Job drawing, mm, ordinate dimensions from the low corner. One solid piece. Round coordinates to 2 decimals unless told otherwise and drop trailing zeros. Loops run counter-clockwise (first coordinate to the right, second up) from the corner with the lowest first, then second, coordinate; pieces in that order, holes last. Notation, with made-up numbers: (-18, -19.5) - (30, -19.5) arc R16 cw to (30, 8.5) - close; hole circle Ø4 at (15, 37.25). An arc over 180 degrees is marked (long way). One line per question, with ' | ' between items. Start each with the question number.
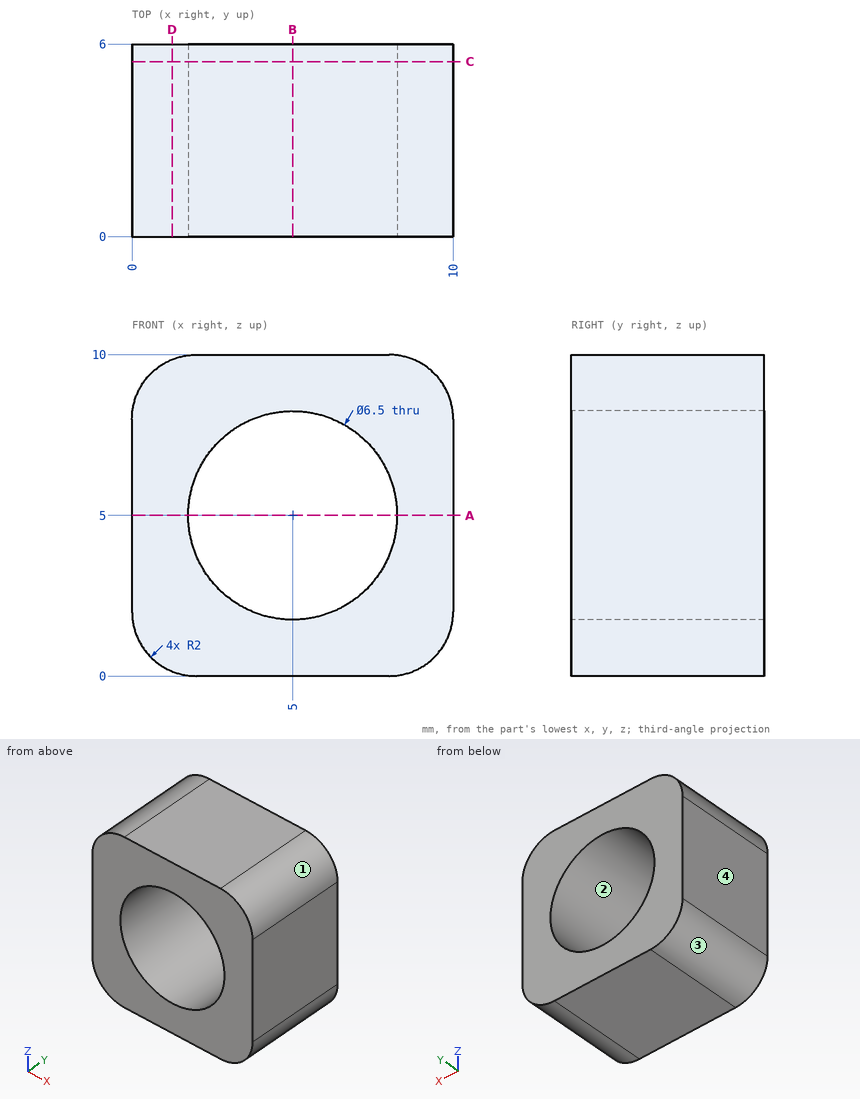
1) Saw through at B-B on x = 5. Write the cut outline in (y, z), and give its area (3 significant figures).
2) Saw through at A-A on z = 5. Write the cut outline in (x, y).
3) Saw through at D-D on x = 1.25. Write the cut outline in (y, z), and give its area (3 significant figures).
4) Saw through at C-C on y = 5.45. Write the cut outline in (x, z), and give its area (3 significant figures).
5) Two-plate mould, pull along Z, no slides. Class the marked faces 1, 2, 3 and 4: +Z half, -Z half, draft (parallel to the pull), parting line (faces both ways), or undercut.
6) Wall check: line 1 (X direction, y = 5.5, z = 5); line 2 (X direction, y = 0.65, z = 3.75). Give the ranges that are in metal, low to high. Write a range as [from, to].
Answer key:
1) outline: (0, 0) - (6, 0) - (6, 1.75) - (0, 1.75) - close; (0, 8.25) - (6, 8.25) - (6, 10) - (0, 10) - close | area: 21.0 mm²
2) outline: (0, 0) - (1.75, 0) - (1.75, 6) - (0, 6) - close; (8.25, 0) - (10, 0) - (10, 6) - (8.25, 6) - close
3) outline: (0, 0.15) - (6, 0.15) - (6, 9.85) - (0, 9.85) - close | area: 58.2 mm²
4) outline: (0, 2) arc R2 ccw to (2, 0) - (8, 0) arc R2 ccw to (10, 2) - (10, 8) arc R2 ccw to (8, 10) - (2, 10) arc R2 ccw to (0, 8) - close; hole circle Ø6.5 at (5, 5) | area: 63.4 mm²
5) face 1: +Z half | face 2: undercut | face 3: -Z half | face 4: draft
6) line 1: [0, 1.75], [8.25, 10] | line 2: [0, 2], [8, 10]
